Verification items for the finished model (mm, model axes). A direction names the side the tool comes from. Give positions to 0.01 mm unless a question says otherwise; leave off trailing zeros. Order: outer loops, then holes, each group sorted by start corner. A loop starts at its lowest first (then second) coordinate and runs counter-clockwise, first axis right, second up. Notation, with made-up numbers: (88, 58) - (119, 58) arc R26 cw to (119, 85) - close; hole circle Ø11 at (64, 12.5). An arc over 180 degrees is marked (long way). Answer as a JSON object with one key per item and string values. Group by question number.
(1) Section check B-B (z = -8). Record the boundary of the cut face in (x, y), then the cut area to 3 significant figures.
(2) Mould release check, pull along Z, two halves, no side actions. Record for faces 6 (the face through (-0.22, -22.307, 10.637)), 7 (the face through (8.284, 5, -2)), 8 (the face through (-0.22, 19.113, -15.666)): +Z half, -Z half, draft (parallel to the pull), parting line (faces both ways), or undercut.
(3) Thickness scan on line 1 (Y direction, x = 2.5, z = -13); line 2 (Z direction, x = 7, y = 14); line 3 (Y direction, x = -4.5, z = 8). Record the ranges inside material, lowest first.
(4) Access from +Z, -Z, +X, -X, +Y, -Y to the whole of each face (thin tool, end or side, straight path). Record for faces 1 (the face through (0.22, 16.399, -8.832)), 2 (the face through (0.22, -4.98, 11.75)), 3 (the face through (-8.284, -5, -2)), 4 (the face through (0.22, -18.77, -0.21)), 5 (the face through (-0.22, -16.59, 18.7)).
(5) Depth check by flat-ended pin: pin 1 Ø0.9 at (x, y) = (5, 0) entering from +Z; pin 2 Ø1.5 at (x, y) = (-5.5, 6.5) entering from -Z; pin 3 Ø16 at (y, z) = (-0.5, 0.5) entering from +X; pin 4 Ø6 at (y, z) = (0, 0) entering from -X. Enter the tip coordinate at first touch or a pass-through.
(6) Section check A-A (z = 14.5). Record the boundary of the cut face in (x, y).
```python
from build123d import *

# Parameters (mm, degrees)
F3_DEPTH = 35
F4_COUNT = 13
F5_R     = 1


with BuildPart() as f1:
    # F0 (on Top) → F1 (revolve)
    with BuildSketch(Plane.XY):
        Polygon((-8.284023578, 9.8717947562), (-8.284023578, 5), (8.284023578, 5), (8.284023578, 9.8717947562), (15.7001973844, 9.8717947562), (15.7001973844, 25), (-15.7001973844, 25), (-15.7001973844, 9.8717947562), align=None)
    revolve(axis=Axis((-9.4565218315, 0, 0), (-1, 0, 0)))

    # F2 (on face) → F3 (cut)
    with BuildSketch(Plane.YZ.offset(15.7001973844)):
        with BuildLine():
            Line((0, 25), (-3.75, 25))
            Line((-3.75, 25), (-1.410776773, 13.3038838649))
            ThreePointArc((-1.410776773, 13.3038838649), (-1.0641850029, 12.7266578587), (-0.4301960973, 12.5))
            Line((-0.4301960973, 12.5), (0, 12.5))
            Line((0, 12.5), (0, 25))
        make_face()
        with BuildLine():
            Line((3.75, 25), (0, 25))
            Line((0, 25), (0, 12.5))
            Line((0, 12.5), (0.4301960973, 12.5))
            ThreePointArc((0.4301960973, 12.5), (1.0641850029, 12.7266578587), (1.410776773, 13.3038838649))
            Line((1.410776773, 13.3038838649), (3.75, 25))
        make_face()
    f3 = extrude(amount=-F3_DEPTH, mode=Mode.SUBTRACT)

    # F4: F3 ×13 about axis
    f4_axis = Axis((15.7001973844, 0, 0), (-1, 0, 0))
    for i in range(1, F4_COUNT):
        add(f3.rotate(f4_axis, i * 360 / F4_COUNT), mode=Mode.SUBTRACT)

    # F5
    f5_edges = [f1.edges().sort_by_distance(p)[0] for p in [
        (0, 14.76231, 20.17608),
        (0, -3.695084, 24.725419),
        (0, 3.695084, 24.725419),
        (0, -14.76231, 20.17608),
        (0, -8.218641, 23.610463),
        (0, -22.447668, 11.004645),
        (0, -18.249574, 17.086633),
        (0, -24.990536, -0.687823),
        (0, -24.09975, 6.648462),
        (0, -21.808374, -12.222718),
        (0, 22.447668, 11.004645),
        (0, 8.218641, 23.610463),
        (0, 24.990536, -0.687823),
        (0, 18.249574, 17.086633),
        (0, 21.808374, -12.222718),
        (0, 24.09975, 6.648462),
        (0, 24.428963, -5.312791),
        (0, 13.630176, -20.957536),
        (0, 19.161796, -16.056948),
        (0, 2.329469, -24.891235),
        (0, 9.504892, -23.122652),
        (0, -9.504892, -23.122652),
        (0, -2.329469, -24.891235),
        (0, -19.161796, -16.056948),
        (0, -13.630176, -20.957536),
        (0, -24.428963, -5.312791),
    ]]
    fillet(f5_edges, radius=F5_R)


solid = f1.part
```
Solutions:
{
 "1": {"outline": "(-15.7, -15.07) - (15.7, -15.07) - (15.7, -5.78) - (8.28, -5.78) - (8.28, 5.78) - (15.7, 5.78) - (15.7, 15.07) - (-15.7, 15.07) - (-15.7, 5.78) - (-8.28, 5.78) - (-8.28, -5.78) - (-15.7, -5.78) - close", "area": "775 mm2"},
 "2": {"face 6": "+Z half", "face 7": "undercut", "face 8": "-Z half"},
 "3": {"line 1": "y = -21.35 to -15.13, -8.99 to -4.75, -1.84 to 1.84, 4.75 to 8.99, 15.13 to 21.35", "line 2": "z = -12.15 to -7.33, -3.58 to 0.16, 3.32 to 7.37, 12.7 to 19.23", "line 3": "y = -23.69 to -15.47, -9.87 to 9.87, 15.47 to 23.69"},
 "4": {"face 1": "+X, -X, +Y", "face 2": "+X, -X", "face 3": "-X", "face 4": "+X, -X, -Y", "face 5": "+Z, +X, -X, -Y"},
 "5": {"pin 1": "stops at z = 12.5", "pin 2": "stops at z = -18.32", "pin 3": "stops at x = 8.28", "pin 4": "passes through"},
 "6": {"outline": "(-15.7, -15.75) - (15.7, -15.75) - (15.7, -10.17) - (-15.7, -10.17) - close; (-15.7, -5.54) - (15.7, -5.54) - (15.7, -1.65) - (-15.7, -1.65) - close; (-15.7, 1.65) - (15.7, 1.65) - (15.7, 5.54) - (-15.7, 5.54) - close; (-15.7, 10.17) - (15.7, 10.17) - (15.7, 15.75) - (-15.7, 15.75) - close"}
}
